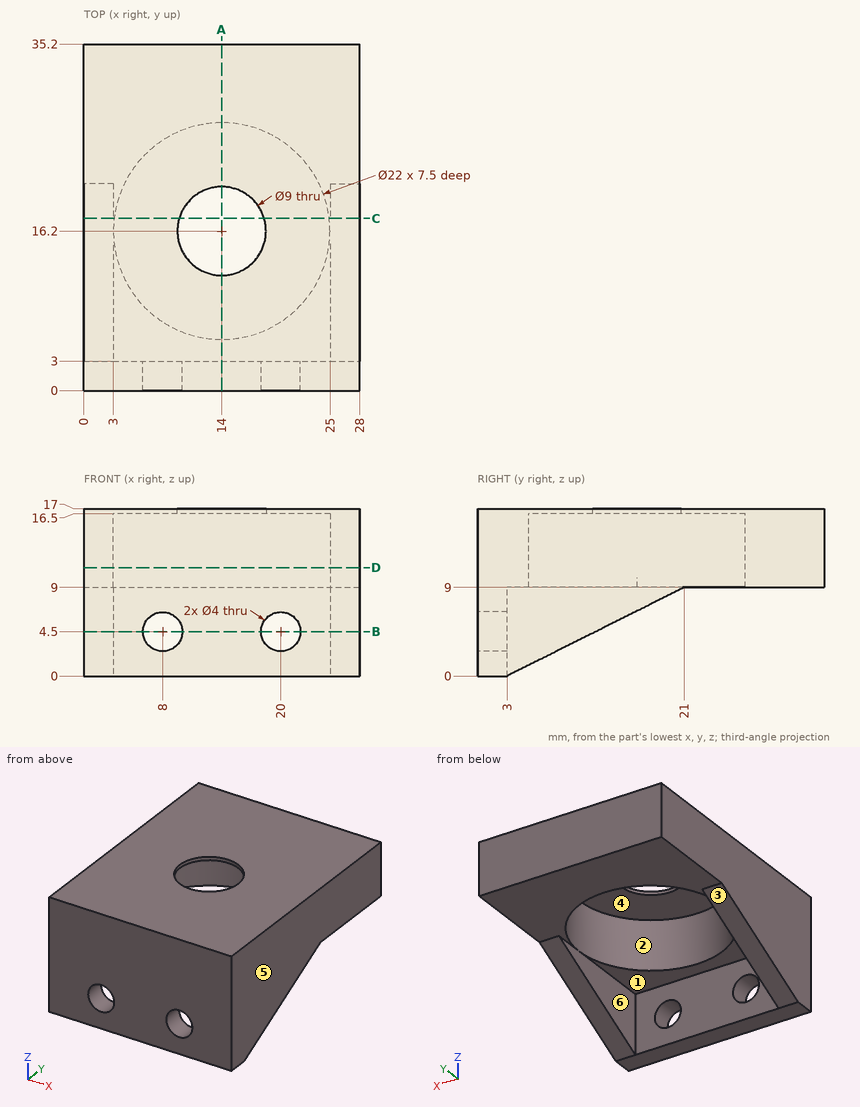
The drawing under review shows one solid part. Ordinate dimensions are in mm from its lowest x, y, z. A direction names the side the tool comes from. Coordinates: 2 decimals unless noted, no trailing zeros. Order: outer loops, then holes, each group sorted by start corner. A loop starts at its lowest first (then second) coordinate and runs counter-clockwise, first axis right, second up. Notation, with made-up numbers: M -39,51.5 L -12,51.5 A33 cw -12,89.5 Z; hole C 84.25,36.5 d6. An arc over 180 degrees is marked long. Use a Markdown table: item, result.
(1) Add section C-C (y = 17.5). Give the boundary of the cut face in (x, z).
Worked answers:
| item | result |
|---|---|
| outline | M 0,7.25 L 3,7.25 L 3,9 L 3.08,9 L 3.08,16.5 L 9.69,16.5 L 9.69,17 L 0,17 Z; M 18.31,16.5 L 24.92,16.5 L 24.92,9 L 25,9 L 25,7.25 L 28,7.25 L 28,17 L 18.31,17 Z |
(2) Add section D-D (z = 11). Give the boundary of the cut face in (x, y).
Worked answers:
| item | result |
|---|---|
| outline | M 0,0 L 28,0 L 28,35.2 L 0,35.2 Z; hole C 14,16.2 d22 |
(3) For P1, Ø3.5, axis at x = 8, z = 4.5, coming from the -Y side; P2, Ø6.5, axis at x = 11.5, y = 11.5, coming from the -Z side; P3, Ø7, axis at x = 12, z = 4.5, coming from the +Y side, all flat-tipped, find the tip position at first contact; note any pin that passes through.
Worked answers:
| item | result |
|---|---|
| P1 | passes through |
| P2 | stops at z = 16.5 |
| P3 | stops at y = 3 |
(4) Wall thickness on probe 1 along Z at (x, y) = (8, 1.5); probe 2 along Y at (x, z) = (14, 13.5); probe 3 along X at (y, z) = (5, 7): over which ranges is each line inside the solid? List them lowest first.
Worked answers:
| item | result |
|---|---|
| probe 1 | z = 0 to 2.5, 6.5 to 17 |
| probe 2 | y = 0 to 5.2, 27.2 to 35.2 |
| probe 3 | x = 0 to 3, 25 to 28 |
(5) For the marked faces 4, 5 and 6, list the 3-axis set-ups (+Z, -Z, +X, -X, +Y, -Y) from which the entire face can be reached by the end or side of a thin tool; tool diameter is ignored.
Worked answers:
| item | result |
|---|---|
| face 4 | -Z |
| face 5 | +Z, -Z, +X, +Y, -Y |
| face 6 | -Z, +Y |
(6) Draft analysis for pull direction Y (two halves, no side actions). For the marked faces 1, 2 and 3, state which applies: released by +Y, released by -Y, zero draft, split by the parting line, or undercut.
Worked answers:
| item | result |
|---|---|
| face 1 | zero draft |
| face 2 | undercut |
| face 3 | released by +Y |
(7) Add section B-B (z = 4.5). Give the boundary of the cut face in (x, y).
Worked answers:
| item | result |
|---|---|
| outline | M 0,0 L 6,0 L 6,3 L 3,3 L 3,12 L 0,12 Z; M 10,0 L 18,0 L 18,3 L 10,3 Z; M 22,0 L 28,0 L 28,12 L 25,12 L 25,3 L 22,3 Z |
(8) Add section A-A (x = 14). Give the boundary of the cut face in (y, z), then the cut area to 3 significant figures.
Worked answers:
| item | result |
|---|---|
| outline | M 0,0 L 3,0 L 3,9 L 5.2,9 L 5.2,16.5 L 11.7,16.5 L 11.7,17 L 0,17 Z; M 20.7,16.5 L 27.2,16.5 L 27.2,9 L 35.2,9 L 35.2,17 L 20.7,17 Z |
| area | 139 mm2 |
